Verification items for the finished model (mm, model axes). Face numbers are marked on the shaded views. A direction names the side the tool comes from. Coordinates: 2 decimals unless noted, no trailing zeros. Write each loop counter-clockwise with the first axis right and the second up, starting at its lowest first coordinate (ties: lowest second). Pieces come first, ordered by that corner, then holes. Notation, with made-up numbers: (80, 66) -> (119, 66) arc R18 ccw to (119, 86) -> close; hole circle Ø11 at (-24, -2). An arc over 180 degrees is marked (long way). Answer in a Markdown table with one row per item.
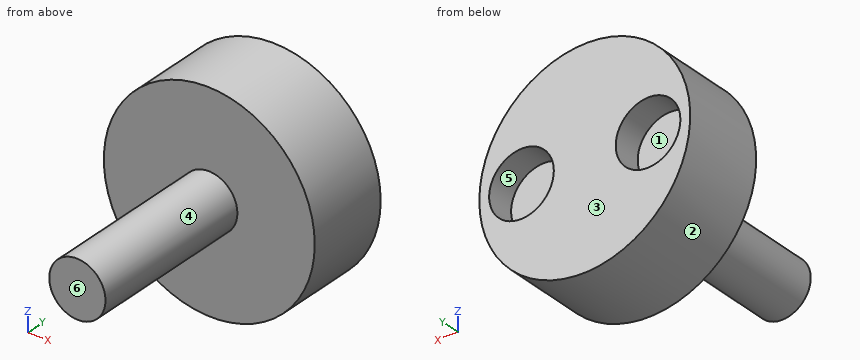
```python
from build123d import *

# Parameters (mm, degrees)
F0_R     = 7.5
F1_DEPTH = 6
F2_R     = 2
F3_DEPTH = 12
F4_R     = 2.3
F5_DEPTH = 2


with BuildPart() as f1:
    # F0 (on Front) → F1 (new body)
    with BuildSketch(Plane.XZ):
        Circle(F0_R)
    extrude(amount=F1_DEPTH)

    # F2 (on face) → F3 (join)
    with BuildSketch(Plane.XZ.offset(6)):
        Circle(F2_R)
    extrude(amount=F3_DEPTH)

    # F4 (on face) → F5 (cut)
    with BuildSketch(Plane(origin=(0, 0, 0), x_dir=(-1, 0, 0), z_dir=(0, 1, 0))):
        with Locations((-4.5, 0)):
            Circle(F4_R)
        with Locations((4.5, 0)):
            Circle(F4_R)
    extrude(amount=-F5_DEPTH, mode=Mode.SUBTRACT)


solid = f1.part
```
1. Sectioned sample at A-A, the plane x = 4.5. Record the cut outline in (y, z).
Findings below:
| item | result |
|---|---|
| outline | (-6, -6) -> (0, -6) -> (0, -2.3) -> (-2, -2.3) -> (-2, 2.3) -> (0, 2.3) -> (0, 6) -> (-6, 6) -> close |
2. Sectioned sample at B-B, the plane z = 0. Record the cut outline in (x, y).
Findings below:
| item | result |
|---|---|
| outline | (-7.5, -6) -> (-2, -6) -> (-2, -18) -> (2, -18) -> (2, -6) -> (7.5, -6) -> (7.5, 0) -> (6.8, 0) -> (6.8, -2) -> (2.2, -2) -> (2.2, 0) -> (-2.2, 0) -> (-2.2, -2) -> (-6.8, -2) -> (-6.8, 0) -> (-7.5, 0) -> close |
3. Go/stop test with flat-tipped pins: pin 1 (6 mm diameter, centred on x = -0.5, y = -7, fed in from +Z); pin 2 (6 mm diameter, centred on y = -6, z = 5.5, fed in from -X); pin 3 (3.5 mm diameter, centred on x = 4.5, z = 0, fed in from +Y); pin 4 (5 mm diameter, centred on x = -5.5, z = -4.5, fed in from -Y). Record where each tip stops, or that it passes through.
Findings below:
| item | result |
|---|---|
| pin 1 | stops at z = 7.5 |
| pin 2 | stops at x = -7.07 |
| pin 3 | stops at y = -2 |
| pin 4 | stops at y = -6 |
4. Sectioned sample at D-D, the plane y = -5. Record the cut outline in (x, z).
Findings below:
| item | result |
|---|---|
| outline | circle Ø15 at (0, 0) |
5. Material ranges on probe 1 along Y at (x, z) = (-4.25, 4); probe 2 along Y at (x, z) = (-6, 1); probe 3 along Z at (x, y) = (-3.75, -1), recorded low to high. Write a range as from..to.
Findings below:
| item | result |
|---|---|
| probe 1 | y = -6..0 |
| probe 2 | y = -6..-2 |
| probe 3 | z = -6.5..-2.17, 2.17..6.5 |
6. Release check for a two-part mould opening along X. For the marked faces 1, 2 and 3 record: released by +X, released by -X, zero draft, split by the parting line, or undercut.
Findings below:
| item | result |
|---|---|
| face 1 | undercut |
| face 2 | split by the parting line |
| face 3 | zero draft |
7. Sectioned sample at C-C, the plane x = 0. Record the cut outline in (y, z), and give its area (3 significant figures).
Findings below:
| item | result |
|---|---|
| outline | (-18, -2) -> (-6, -2) -> (-6, -7.5) -> (0, -7.5) -> (0, 7.5) -> (-6, 7.5) -> (-6, 2) -> (-18, 2) -> close |
| area | 138 mm² |
8. Access from +Z, -Z, +X, -X, +Y, -Y to the whole of each face (thin tool, end or side, straight path). Record for the marked faces 4, 5 and 6.
Findings below:
| item | result |
|---|---|
| face 4 | -Y |
| face 5 | +Y |
| face 6 | +Z, -Z, +X, -X, -Y |
